```python
from build123d import *

# Parameters (mm, degrees)
SKETCH_W        = 18.6
SKETCH_H        = 93
PAD_DEPTH       = 6
SKETCH001_W     = 3
SKETCH001_H     = 6
POCKET_DEPTH    = 6
POCKET001_DEPTH = 8
PAD001_DEPTH    = 2
SKETCH004_R     = 1.551846
SKETCH004_R_2   = 1.552141
POCKET002_DEPTH = 55
SKETCH005_W     = 80
SKETCH005_H     = 40
PAD002_DEPTH    = 2.5


with BuildPart() as part:
    # Sketch → Pad (new body)
    with BuildSketch(Plane.XY):
        Rectangle(SKETCH_W, SKETCH_H)
    extrude(amount=-PAD_DEPTH)

    # Sketch001 (on Face5 of Pad) → Pocket (cut)
    with BuildSketch(Plane.XY):
        Rectangle(SKETCH001_W, SKETCH001_H)
    extrude(amount=-POCKET_DEPTH, mode=Mode.SUBTRACT)

    # Sketch002 (on Face4 of Pocket) → Pocket001 (cut)
    with BuildSketch(Plane.XY):
        with BuildLine():
            ThreePointArc((-2.5, -42), (0, -44.5), (2.5, -42))
            Line((2.5, -42), (2.5, -32))
            ThreePointArc((2.5, -32), (0, -29.5), (-2.5, -32))
            Line((-2.5, -42), (-2.5, -32))
        make_face()
        with BuildLine():
            ThreePointArc((-8.5, -42), (-6, -44.5), (-3.5, -42))
            Line((-3.5, -42), (-3.5, -32))
            ThreePointArc((-3.5, -32), (-6, -29.5), (-8.5, -32))
            Line((-8.5, -42), (-8.5, -32))
        make_face()
        with BuildLine():
            ThreePointArc((3.5, -42), (6, -44.5), (8.5, -42))
            Line((8.5, -42), (8.5, -32))
            ThreePointArc((8.5, -32), (6, -29.5), (3.5, -32))
            Line((3.5, -42), (3.5, -32))
        make_face()
        with BuildLine():
            ThreePointArc((-2.487782, -26), (0.012218, -28.5), (2.512218, -26))
            Line((2.512218, -26), (2.512218, -16))
            ThreePointArc((2.512218, -16), (0.012218, -13.5), (-2.487782, -16))
            Line((-2.487782, -26), (-2.487782, -16))
        make_face()
        with BuildLine():
            ThreePointArc((-8.496945, -26), (-6, -28.496945), (-3.503055, -26))
            Line((-3.503055, -26), (-3.503055, 8))
            ThreePointArc((-3.503055, 8), (-6, 10.496945), (-8.496945, 8))
            Line((-8.496945, -26), (-8.496945, 8))
        make_face()
        with BuildLine():
            ThreePointArc((3.503055, -26), (6, -28.496945), (8.496945, -26))
            Line((8.496945, -26), (8.496945, 8))
            ThreePointArc((8.496945, 8), (6, 10.496945), (3.503055, 8))
            Line((3.503055, -26), (3.503055, 8))
        make_face()
        with BuildLine():
            ThreePointArc((2.5, 42), (0, 44.5), (-2.5, 42))
            Line((-2.5, 42), (-2.5, 32))
            ThreePointArc((-2.5, 32), (0, 29.5), (2.5, 32))
            Line((2.5, 42), (2.5, 32))
        make_face()
        with BuildLine():
            ThreePointArc((-3.5, 42), (-6, 44.5), (-8.5, 42))
            Line((-8.5, 42), (-8.5, 32))
            ThreePointArc((-8.5, 32), (-6, 29.5), (-3.5, 32))
            Line((-3.5, 42), (-3.5, 32))
        make_face()
        with BuildLine():
            ThreePointArc((8.5, 42), (6, 44.5), (3.5, 42))
            Line((3.5, 42), (3.5, 32))
            ThreePointArc((3.5, 32), (6, 29.5), (8.5, 32))
            Line((8.5, 42), (8.5, 32))
        make_face()
        with BuildLine():
            ThreePointArc((2.512218, 26), (0.012218, 28.5), (-2.487782, 26))
            Line((-2.487782, 26), (-2.487782, 16))
            ThreePointArc((-2.487782, 16), (0.012218, 13.5), (2.512218, 16))
            Line((2.512218, 26), (2.512218, 16))
        make_face()
        with BuildLine():
            ThreePointArc((-3.487782, 26), (-5.987782, 28.5), (-8.487782, 26))
            Line((-8.487782, 26), (-8.487782, 16))
            ThreePointArc((-8.487782, 16), (-5.987782, 13.5), (-3.487782, 16))
            Line((-3.487782, 26), (-3.487782, 16))
        make_face()
        with BuildLine():
            ThreePointArc((8.496945, 26), (6, 28.496945), (3.503055, 26))
            Line((3.503055, 26), (3.503055, 16))
            ThreePointArc((3.503055, 16), (6, 13.503055), (8.496945, 16))
            Line((8.496945, 26), (8.496945, 16))
        make_face()
    extrude(amount=-POCKET001_DEPTH, mode=Mode.SUBTRACT)

    # Sketch003 (on Face3 of Pocket001) → Pad001 (join)
    with BuildSketch(Plane.YZ.offset(9.3)):
        Polygon((-24, -6), (-24, 0), (-10.960923, 6), (-10.960923, 37), (-3, 37), (-3, 6), (3, 6), (3, 37), (10.971753, 37), (10.971753, 6), (24, 0), (24, -6), align=None)
    extrude(amount=PAD001_DEPTH)

    # Sketch004 → Pocket002 (cut)
    with BuildSketch(Plane.YZ.offset(11.3)):
        with Locations((-8.8, 31.464135)):
            Circle(SKETCH004_R)
        with Locations((8.8, 31.541361)):
            Circle(SKETCH004_R_2)
    extrude(amount=-POCKET002_DEPTH, mode=Mode.SUBTRACT)

    # Sketch005 (on Face5 of Pocket002) → Pad002 (join)
    with BuildSketch(Plane(origin=(0, 0, -6), x_dir=(1, 0, 0), z_dir=(0, 0, -1))):
        with Locations((0, 60)):
            Rectangle(SKETCH005_W, SKETCH005_H)
    extrude(amount=-PAD002_DEPTH)


solid = part.part
```
Part model, mm, in its own coordinate system. A direction names the side the tool comes from. Give positions to 0.01 mm unless a question says otherwise; leave off trailing zeros. Write each loop counter-clockwise with the first axis right and the second up, starting at its lowest first coordinate (ties: lowest second). Pieces come first, ordered by that corner, then holes. Notation, with made-up numbers: M 79,57.25 L 104,57.25 A22 cw 104,89.25 Z; hole C 89,3 d5. An arc over 180 degrees is marked long. Use CSV: the item, a comma, the result in double quotes.
Item 1: Slice it at A-A on y = -8.8. Write the cut outline in (x, z), plus the area to 3 significant figures.
Taken from the geometry:
outline,"M -9.3,-6 L -8.5,-6 L -8.5,0 L -9.3,0 Z; M -3.5,-6 L 3.5,-6 L 3.5,0 L -3.5,0 Z; M 8.5,-6 L 11.3,-6 L 11.3,29.91 L 9.3,29.91 L 9.3,0 L 8.5,0 Z; M 9.3,33.02 L 11.3,33.02 L 11.3,37 L 9.3,37 Z"
area,"131 mm²"
Item 2: Drill centre lines: probe 1 along Z at (x, y) = (10.8, -8.8); probe 2 along Y at (x, z) = (11, 12); probe 3 along Z at (x, y) = (10.5, 8.8). Where is each one in solid material? Low to high.
Taken from the geometry:
probe 1,"z = -6 to 29.91, 33.02 to 37"
probe 2,"y = -10.96 to -3, 3 to 10.97"
probe 3,"z = -6 to 29.99, 33.09 to 37"
Item 3: Slice it at B-B on x = 6. Write the cut outline in (y, z).
Taken from the geometry:
outline,"M -80,-6 L -40,-6 L -40,-3.5 L -44.5,-3.5 L -44.5,0 L -46.5,0 L -46.5,-3.5 L -80,-3.5 Z; M -29.5,-6 L -28.5,-6 L -28.5,0 L -29.5,0 Z; M 10.5,-6 L 13.5,-6 L 13.5,0 L 10.5,0 Z; M 28.5,-6 L 29.5,-6 L 29.5,0 L 28.5,0 Z; M 44.5,-6 L 46.5,-6 L 46.5,0 L 44.5,0 Z"
Item 4: Pull direction Y, two halves, no side cores. Call faces 1 (the face through (10.314, -9.944, 32.513)), 2 (the face through (-1, -60, -6)), 3 (the face through (2.5, 37, -3)), 4 (the face through (10.286, 17.395, 3.042)): +Y half, -Y half, draft (parallel to the pull), parting line (faces both ways), or undercut.
Taken from the geometry:
face 1,"undercut"
face 2,"draft"
face 3,"undercut"
face 4,"+Y half"
Item 5: Slice it at C-C on z = 8. Write the cut outline in (x, y), plus the area to 3 significant figures.
Taken from the geometry:
outline,"M 9.3,-10.96 L 11.3,-10.96 L 11.3,-3 L 9.3,-3 Z; M 9.3,3 L 11.3,3 L 11.3,10.97 L 9.3,10.97 Z"
area,"31.9 mm²"
Item 6: Pin check, flat tips, straight feed: P1, Ø6.5, axis at y = 20, z = -3, coming from the +X side; P2, Ø1, axis at x = 10.5, y = -0.5, coming from the +Z side; P3, Ø6.5, axis at y = 38, z = -4, coming from the +X side; P4, Ø1, axis at x = 12, y = -9.5, coming from the -Z side. Stop position of each tip, or through.
Taken from the geometry:
P1,"stops at x = 11.3"
P2,"stops at z = 6"
P3,"stops at x = 9.3"
P4,"passes through"
Item 7: Which spindle directions (+Z, -Z, +X, -X, +Y, -Y) get a long thin tool onto all of the face, cutting with end or side? Do faces 5 (the face through (-25, -40, -5)), 6 (the face through (-6, -42, -3.5)), 7 (the face through (0.1, -29.5, -3)). Say none if no direction does.
Taken from the geometry:
face 5,"+Z, -Z, -X, +Y"
face 6,"+Z"
face 7,"+Z, -Z"
Item 8: Slice it at D-D on x = 15. Write the cut outline in (y, z), plus the area to 3 significant figures.
Taken from the geometry:
outline,"M -80,-6 L -40,-6 L -40,-3.5 L -80,-3.5 Z"
area,"100 mm²"
